Source: CAD feature listing. Evaluate the final solid. Frame: model axes, mm. A direction names the side the tool comes from. Coordinates: 2 decimals unless noted, no trailing zeros. Loops run counter-clockwise (first coordinate to the right, second up) from the corner with the lowest first, then second, coordinate; pieces in that order, holes last.
Item 1: Pin query (flat end, axial travel): pin 1 Ø6.5 at (y, z) = (195, 200.75) entering from +X; pin 2 Ø12 at (y, z) = (176, 25.5) entering from -X; pin 3 Ø6 at (x, z) = (-32, 78.5) entering from +Y. Return the tip coordinate at first contact, or that it passes through.
Item 2: Section query A-A, the plane z = -244. Return the cut outline in (x, y).
Item 3: Reachability of faces 1 (the flat face through (-19, 1, -6)), 2 (the flat face through (0.3, 112, -421.5)) from +Z, -Z, +X, -X, +Y, -Y: full face, straight path, thin tool, end or side. Return the list, or none.
Item 4: Line query: probe 1 along Y at (x, z) = (0.3, -401.5); probe 2 along X at (y, z) = (202, -370). Output: solid intervals per line, ascending.
Item 5: Section query B-B, the plane x = -13.5. Return the cut outline in (y, z), then the cut area to 3 significant figures.
```python
from build123d import *

# Parameters (mm, degrees)
SKETCH2_W                    = 1
SKETCH2_H                    = 225
BASE_FLANGE1_DEPTH           = 421.5
EDGE_FLANGE1_STRIP_W         = 8
EDGE_FLANGE1_STRIP_H         = 1
EDGE_FLANGE1_STRIP_CUT_DEPTH = 843
EDGE_FLANGE1_DEPTH           = 843
CRVPATTERN1_COUNT            = 9
CRVPATTERN1_PITCH            = 100.375
FILLET1_R                    = 2


# Sheet-metal steps are written as plain solids
with BuildPart() as part:
    # Sketch2 → Base-Flange1 (new, symmetric)
    with BuildSketch(Plane.XY):
        with Locations((0.5, 112.5)):
            Rectangle(SKETCH2_W, SKETCH2_H)
    extrude(amount=BASE_FLANGE1_DEPTH, both=True)

    # Edge-Flange1 strip (across the edge) → Edge-Flange1 strip cut (cut)
    with BuildSketch(Plane(origin=(0, 0, -421.5), x_dir=(0, 1, 0), z_dir=(0, 0, 1))):
        with Locations((-1, -0.5)):
            Rectangle(EDGE_FLANGE1_STRIP_W, EDGE_FLANGE1_STRIP_H)
    extrude(amount=EDGE_FLANGE1_STRIP_CUT_DEPTH, mode=Mode.SUBTRACT)

    # Edge-Flange1 section (across the edge) → Edge-Flange1 (add)
    with BuildSketch(Plane(origin=(0, 0, -421.5), x_dir=(0, 1, 0), z_dir=(0, 0, 1))):
        with BuildLine():
            Line((0, 2), (0, 36))
            Line((0, 36), (1, 36))
            Line((1, 36), (1, 2))
            ThreePointArc((1, 2), (1.585786438, 0.585786438), (3, 0))
            Line((3, 0), (3, -1))
            ThreePointArc((3, -1), (0.878679656, -0.121320344), (0, 2))
        make_face()
    extrude(amount=EDGE_FLANGE1_DEPTH)

    # Sketch8 → M5 Clearance Hole1 (revolve, cut)
    with BuildSketch(Plane(origin=(0, 195, -401.5), x_dir=(0, 0, 1), z_dir=(0, 1, 0))):
        Polygon((0, 0), (0, 1), (2.75, 1), (2.75, 0.025), (2.775, 0), align=None)
    m5_clearance_hole1 = revolve(axis=Axis((-6.35, 195, -401.5), (1, 0, 0)), mode=Mode.SUBTRACT)

    # CrvPattern1: M5 Clearance Hole1 ×9
    with Locations(*[(0, 0, i * CRVPATTERN1_PITCH) for i in range(1, CRVPATTERN1_COUNT)]):
        add(m5_clearance_hole1, mode=Mode.SUBTRACT)

    # Fillet1
    fillet1_edges = [part.edges().sort_by_distance(p)[0] for p in [
        (-36, 0.5, -421.5),
        (-36, 0.5, 421.5),
        (0.5, 225, -421.5),
        (0.5, 225, 421.5),
    ]]
    fillet(fillet1_edges, radius=FILLET1_R)


solid = part.part
```
Verdict:
1. pin 1: stops at x = 1
1. pin 2: stops at x = 0
1. pin 3: stops at y = 1
2. outline: (-36, 0) - (-2, 0) arc R3 ccw to (1, 3) - (1, 225) - (0, 225) - (0, 3) arc R2 cw to (-2, 1) - (-36, 1) - close
3. face 1: +Z, -Z, -X, +Y
3. face 2: -Z, +X, -X, +Y, -Y
4. probe 1: y = 1.07 to 192.25, 197.75 to 225
4. probe 2: x = 0 to 1
5. outline: (0, -421.5) - (1, -421.5) - (1, 421.5) - (0, 421.5) - close
5. area: 843 mm2
